Design review of the part shown in the three views and the two pictorial views. Dimensions are in mm from the part's minimum x, y and z. A direction names the side the tool comes from. Round coordinates to 2 decimals unless told otherwise and drop trailing zeros. Loops run counter-clockwise (first coordinate to the right, second up) from the corner with the lowest first, then second, coordinate; pieces in that order, holes last.
1) Insertion check: pin 1 (4 mm diameter, centred on x = 63, y = 13, fed in from -Z); pin 2 (1.5 mm diameter, centred on x = 36.5, y = 4, fed in from -Z); pin 3 (3 mm diameter, centred on y = 7, z = 2, fed in from -X); pin 4 (3 mm diameter, centred on y = 8.5, z = 14, fed in from -X). Each pin has a flat end and moves straight along its axis. Give the tip position at first contact, or say it passes through.
2) Wall thickness on L1, parallel to X at y = 11.5, z = 16.75; L2, parallel to Z at x = 37.5, y = 9.5; L3, parallel to Y at x = 68, z = 10: over which ranges is each line inside the solid? List them lowest first.
3) Tool access review of the marked faces 1, 2 and 3: name each direction out of +Z, -Z, +X, -X, +Y, -Y from which nothing blocks a thin tool from reaching the whole face with its end or side.
4) Take a section at A-A (z = 10). State the section outline as (x, y) points.
5) Take a section at D-D (x = 24). State the section outline as (y, z) points, then the cut area to 3 significant figures.
6) Take a section at C-C (x = 7). State the section outline as (y, z) points.
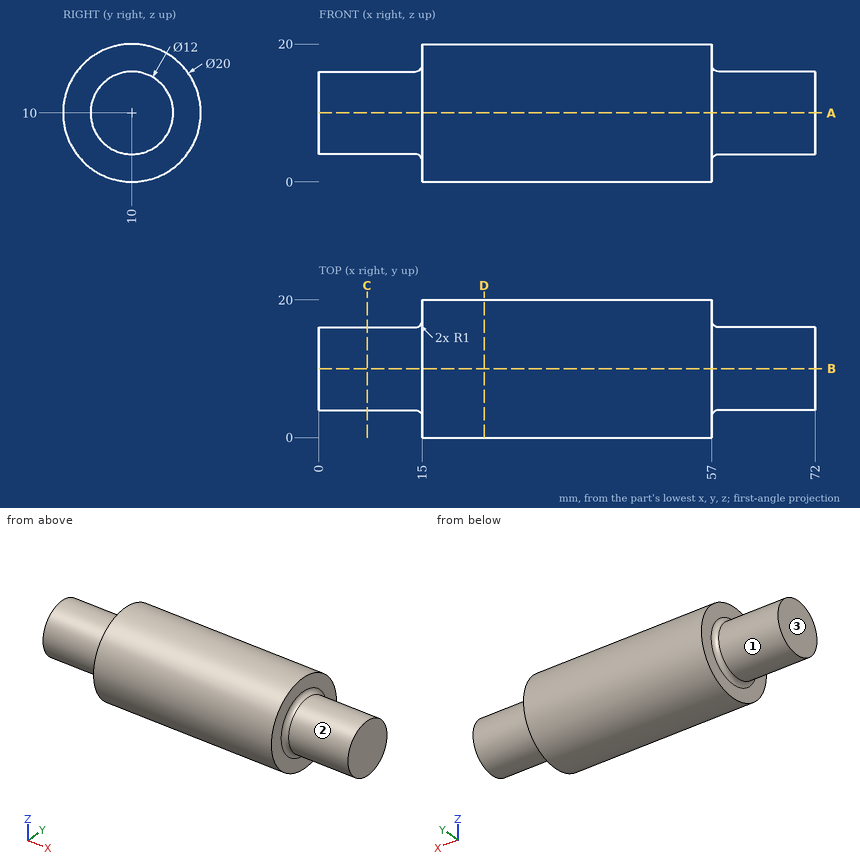
Response:
1. pin 1: stops at z = 4.08
1. pin 2: stops at z = 1.49
1. pin 3: stops at x = 15
1. pin 4: stops at x = 0
2. L1: x = 15 to 57
2. L2: z = 0.01 to 19.99
2. L3: y = 4 to 16
3. face 1: -X
3. face 2: +X
3. face 3: +Z, -Z, -X, +Y, -Y
4. outline: (0, 4) - (14, 4) arc R1 cw to (15, 3) - (15, 0) - (57, 0) - (57, 3) arc R1 cw to (58, 4) - (72, 4) - (72, 16) - (58, 16) arc R1 cw to (57, 17) - (57, 20) - (15, 20) - (15, 17) arc R1 cw to (14, 16) - (0, 16) - close
5. outline: circle Ø20 at (10, 10)
5. area: 314 mm2
6. outline: circle Ø12 at (10, 10)
